Can you work these out from the model? Positions are in its coordinate system, mm. Face numbers are marked on the shaded views. A direction names the side the tool comes from. Round coordinates to 2 decimals unless told otherwise and drop trailing zeros. Loops run counter-clockwise (first coordinate to the right, second up) from the corner with the lowest first, then second, coordinate; pieces in that order, holes last. Notation, with made-up numbers: (59.25, 59) -> (105.25, 59) arc R20 ccw to (105.25, 63) -> close; hole circle Ø5 at (73.25, -27). An arc over 180 degrees is marked (long way). Answer as a JSON object with one key per item and string values.
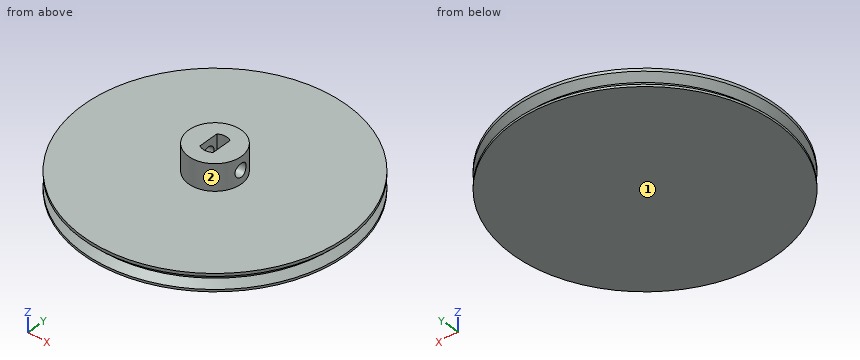
```python
from build123d import *

# Parameters (mm, degrees)
F0_R     = 30
F1_DEPTH = 4
F2_R     = 6
F3_DEPTH = 6
F4_R     = 1.5
F5_DEPTH = 12.3


with BuildPart() as f1:
    # F0 (on Top) → F1 (new body)
    with BuildSketch(Plane.XY):
        Circle(F0_R)
    extrude(amount=F1_DEPTH)

    # F2 (on face) → F3 (join)
    with BuildSketch(Plane.XY.offset(4)):
        Circle(F2_R)
        with BuildLine():
            Line((1.5, 2.3), (1.5, -2.3))
            ThreePointArc((1.5, -2.3), (0, -2.745906), (-1.5, -2.3))
            Line((-1.5, -2.3), (-1.5, 2.3))
            ThreePointArc((-1.5, 2.3), (0, 2.745906), (1.5, 2.3))
        make_face(mode=Mode.SUBTRACT)
    extrude(amount=F3_DEPTH)

    # F4 (on Right) → F5 (cut, symmetric)
    with BuildSketch(Plane.YZ):
        with Locations((0, 7)):
            Circle(F4_R)
    extrude(amount=F5_DEPTH, both=True, mode=Mode.SUBTRACT)

    # F6 (on Front) → F7 (revolve, cut)
    with BuildSketch(Plane.XZ):
        Polygon((-30, 3.33949), (-30, 0.511062), (-28.585786, 1.925276), align=None)
    revolve(axis=Axis((0, 0, 6.11444), (0, 0, -1)), mode=Mode.SUBTRACT)


solid = f1.part
```
Q1. I want a section at B-B, the plane z = 7. Write out the boundary of the cut face in (x, y).
Determined:
{"outline": "(-5.81, -1.5) arc R6 ccw to (5.81, -1.5) -> (1.5, -1.5) -> (1.5, -2.3) arc R2.75 cw to (-1.5, -2.3) -> (-1.5, -1.5) -> close; (-5.81, 1.5) -> (-1.5, 1.5) -> (-1.5, 2.3) arc R2.75 cw to (1.5, 2.3) -> (1.5, 1.5) -> (5.81, 1.5) arc R6 ccw to start"}
Q2. I'm going to push flat-ended pins straight in: pin 1 (8 mm diameter, centred on x = 21.5, y = 13.5, fed in from -Z); pin 2 (5 mm diameter, centred on y = -1, z = 7.5, fed in from +X); pin 3 (2 mm diameter, centred on y = 8.5, z = 7.5, fed in from +X); pin 4 (1 mm diameter, centred on x = 3.5, z = 7, fed in from -Y). Where does each tip first touch, or does it pass through?
Determined:
{"pin 1": "z = 0", "pin 2": "x = 6", "pin 3": "through", "pin 4": "y = -5.2"}
Q3. On a 3-axis mill with a long thin cutter (end or side, diameter ignored), from which of +Z, -Z, +X, -X, +Y, -Y can I reach the whole of each face in a straight line? I mean the marked faces 1 and 2. Say none if no direction works.
Determined:
{"face 1": "-Z, +X, -X, +Y, -Y", "face 2": "+Z"}
Q4. If I drill on L1, parallel to Z at x = 4.4, y = 0; L2, parallel to Z at x = 25, y = -7.5; L3, parallel to Y at x = -0.5, z = 7.25, over which ranges is the centre line in solid material (lowest first)? Write a range as [from, to].
Determined:
{"L1": "[0, 5.5], [8.5, 10]", "L2": "[0, 4]", "L3": "[-5.98, -2.7], [2.7, 5.98]"}
Q5. I want a section at A-A, the plane y = 0. Write out the boundary of the cut face in (x, z).
Determined:
{"outline": "(-30, 0) -> (30, 0) -> (30, 0.51) -> (28.59, 1.93) -> (30, 3.34) -> (30, 4) -> (6, 4) -> (6, 5.5) -> (1.5, 5.5) -> (1.5, 4) -> (-1.5, 4) -> (-1.5, 5.5) -> (-6, 5.5) -> (-6, 4) -> (-30, 4) -> (-30, 3.34) -> (-28.59, 1.93) -> (-30, 0.51) -> close; (-6, 8.5) -> (-1.5, 8.5) -> (-1.5, 10) -> (-6, 10) -> close; (1.5, 8.5) -> (6, 8.5) -> (6, 10) -> (1.5, 10) -> close"}
Q6. I want a section at C-C, the plane x = 0. Write out the boundary of the cut face in (y, z).
Determined:
{"outline": "(-30, 0) -> (30, 0) -> (30, 0.51) -> (28.59, 1.93) -> (30, 3.34) -> (30, 4) -> (6, 4) -> (6, 10) -> (2.75, 10) -> (2.75, 4) -> (-2.75, 4) -> (-2.75, 10) -> (-6, 10) -> (-6, 4) -> (-30, 4) -> (-30, 3.34) -> (-28.59, 1.93) -> (-30, 0.51) -> close"}
